Can you work these out from the model? Positions are in its coordinate system, mm. A direction names the side the tool comes from. Round coordinates to 2 decimals unless told otherwise and drop trailing zeros. Order: outer loops, then holes, each group sorted by start corner. A loop starts at its lowest first (then second) coordinate and runs counter-clockwise, first axis right, second up. Notation, with made-up numbers: M 6.25,48 L 62.25,48 A33 ccw 62.25,84 Z; hole C -23.75,20 d8. An arc over 180 degrees is marked long. Answer as a JSON object with one key per item and string values. Group by question number.
```python
from build123d import *

# Parameters (mm, degrees)
SKETCH1_W           = 1828.8
SKETCH1_H           = 762
BOSS_EXTRUDE1_DEPTH = 25.4
BOSS_EXTRUDE2_DEPTH = 76.2
CUT_EXTRUDE2_DEPTH  = 1892.621171867
CUT_EXTRUDE3_DEPTH  = 116.84
CUT_EXTRUDE4_DEPTH  = 116.84


with BuildPart() as part:
    # Sketch1 → Boss-Extrude1 (new body)
    with BuildSketch(Plane.XY):
        with Locations((875.396405659, 338.441890904)):
            Rectangle(SKETCH1_W, SKETCH1_H)
    extrude(amount=BOSS_EXTRUDE1_DEPTH)

    # Sketch4 → Boss-Extrude2 (add)
    with BuildSketch(Plane.XY.offset(25.4)):
        Polygon((341.996405659, 116.191890904), (291.196405659, 116.191890904), (291.196405659, 103.491890904), (392.796405659, 103.491890904), (392.796405659, 116.191890904), align=None)
        Polygon((874.604865323, 116.863799968), (823.804865323, 116.863799968), (823.804865323, 104.163799968), (925.404865323, 104.163799968), (925.404865323, 116.863799968), align=None)
        Polygon((1408.796405659, 115.67295816), (1357.996405659, 115.67295816), (1357.996405659, 104.010823647), (1459.596405659, 104.010823647), (1459.596405659, 115.67295816), align=None)
    extrude(amount=BOSS_EXTRUDE2_DEPTH)

    # Sketch6 → Cut-Extrude2 (cut, through all)
    with BuildSketch(Plane(origin=(0, 115.67295816, 0), x_dir=(1, 0, 0), z_dir=(0, 1, 0))):
        with BuildLine():
            Line((1459.596405659, -25.4), (1459.596405659, -101.6))
            Line((1459.596405659, -101.6), (1357.996405659, -101.6))
            Line((1357.996405659, -101.6), (1357.996405659, -25.4))
            ThreePointArc((1357.996405659, -25.4), (1408.796405659, -76.2), (1459.596405659, -25.4))
        make_face()
    extrude(amount=-CUT_EXTRUDE2_DEPTH, mode=Mode.SUBTRACT)

    # Sketch7 → Cut-Extrude3 (cut)
    with BuildSketch(Plane(origin=(0, 116.863799968, 0), x_dir=(1, 0, 0), z_dir=(0, 1, 0))):
        with BuildLine():
            Line((925.404865323, -25.4), (925.404865323, -101.6))
            Line((925.404865323, -101.6), (823.804865323, -101.6))
            Line((823.804865323, -101.6), (823.804865323, -25.4))
            ThreePointArc((823.804865323, -25.4), (874.604865323, -76.2), (925.404865323, -25.4))
        make_face()
    extrude(amount=-CUT_EXTRUDE3_DEPTH, mode=Mode.SUBTRACT)

    # Sketch8 → Cut-Extrude4 (cut)
    with BuildSketch(Plane(origin=(0, 116.191890904, 0), x_dir=(1, 0, 0), z_dir=(0, 1, 0))):
        with BuildLine():
            Line((392.796405659, -25.4), (392.796405659, -101.6))
            Line((392.796405659, -101.6), (291.196405659, -101.6))
            Line((291.196405659, -101.6), (291.196405659, -25.4))
            ThreePointArc((291.196405659, -25.4), (341.996405659, -76.2), (392.796405659, -25.4))
        make_face()
    extrude(amount=-CUT_EXTRUDE4_DEPTH, mode=Mode.SUBTRACT)


solid = part.part
```
1) If we section it at B-B on x = 1510: Write out the boundary of the cut face in (y, z), plus the area to 3 significant figures.
2) Which directions (+Z, -Z, +X, -X, +Y, -Y) give clear straight access to the entire face, cutting with the end or side of a thin tool? Please do faces 4 (the face through (341, 103.492, 45)), 5 (the face through (875, 116.864, 45)), 6 (the face through (1410, 115.673, 45)), 7 (the face through (1407.679, 109.924, 76.188)).
3) If we section it at A-A on z = 50.5: Write out the boundary of the cut face in (x, y), plus the area to 3 significant figures.
4) If we section it at C-C on y = 267: Write out the boundary of the cut face in (x, z), plus the area to 3 significant figures.
5) We'd pull the mould along X, two halves only. Please class faces 1 (the face through (1408, 104.011, 45)), 2 (the face through (873.488, 110.603, 76.188)), 3 (the face through (340.879, 109.931, 76.188)): +X half, -X half, draft (parallel to the pull), parting line (faces both ways), or undercut.
6) For pin 1 (15 mm diameter, centred on x = 865, z = 38.5, fed in from +Y); pin 2 (1.5 mm diameter, centred on x = 550, y = 246.5, fed in from +Z); pin 3 (15 mm diameter, centred on x = 880, z = 45.5, fed in from -Y), each with a flat end and sliding along its axis, tell me the tip position at first contact or that it passes through.
7) I need wall thicknesses on line 1 along Z through (x, y) = (824.5, 396.5); line 2 along Y through (x, z) = (1441.5, 50). Which ranges of each line are inside material? Lowest first, please.
Findings:
{
 "1": {"outline": "M -42.56,0 L 719.44,0 L 719.44,25.4 L -42.56,25.4 Z", "area": "19,400 mm^2"},
 "2": {"face 4": "+Z, +X, -X, -Y", "face 5": "+Z, +X, -X, +Y", "face 6": "+Z, +X, +Y", "face 7": "+Z, +Y, -Y"},
 "3": {"outline": "M 297.83,103.49 L 386.16,103.49 L 386.16,116.19 L 297.83,116.19 Z; M 830.44,104.16 L 918.77,104.16 L 918.77,116.86 L 830.44,116.86 Z; M 1364.63,104.01 L 1452.96,104.01 L 1452.96,115.67 L 1364.63,115.67 Z", "area": "3,270 mm^2"},
 "4": {"outline": "M -39,0 L 1789.8,0 L 1789.8,25.4 L -39,25.4 Z", "area": "46,500 mm^2"},
 "5": {"face 1": "draft", "face 2": "undercut", "face 3": "undercut"},
 "6": {"pin 1": "stops at y = 116.86", "pin 2": "stops at z = 25.4", "pin 3": "stops at y = 104.16"},
 "7": {"line 1": "z = 0 to 25.4", "line 2": "y = 104.01 to 115.67"}
}
